from build123d import *

# Parameters (mm, degrees)
BOSS_EXTRUDE1_DEPTH = 6
SKETCH2_R           = 2.5
SKETCH2_R_2         = 12.5
SKETCH2_R_3         = 1.5
CUT_EXTRUDE1_DEPTH  = 96.876222287


with BuildPart() as part:
    # Sketch1 → Boss-Extrude1 (new body)
    with BuildSketch(Plane(origin=(0, 0, 0), x_dir=(1, 0, 0), z_dir=(0, 1, 0))):
        Polygon((0, 0), (-52.5, 0), (-52.5, 80), (52.5, 80), (52.5, 0), align=None)
    extrude(amount=BOSS_EXTRUDE1_DEPTH)

    # Sketch2 → Cut-Extrude1 (cut, through all)
    with BuildSketch(Plane(origin=(0, 6, 0), x_dir=(1, 0, 0), z_dir=(0, 1, 0))):
        with Locations(Location((-42.5, 70, 0), (0, 0, 270))):
            Circle(SKETCH2_R)
        with Locations(Location((42.5, 70, 0), (0, 0, 270))):
            Circle(SKETCH2_R)
        with Locations(Location((42.5, 10, 0), (0, 0, 270))):
            Circle(SKETCH2_R)
        with Locations(Location((0, 10, 0), (0, 0, 270))):
            Circle(SKETCH2_R)
        with Locations(Location((-42.5, 10, 0), (0, 0, 270))):
            Circle(SKETCH2_R)
        with Locations(Location((0, 41, 0), (0, 0, 270))):
            Circle(SKETCH2_R_2)
        with Locations(Location((-15.5, 56.5, 0), (0, 0, 270))):
            Circle(SKETCH2_R_3)
        with Locations(Location((15.5, 56.5, 0), (0, 0, 270))):
            Circle(SKETCH2_R_3)
        with Locations(Location((-15.5, 25.5, 0), (0, 0, 270))):
            Circle(SKETCH2_R_3)
        with Locations(Location((15.5, 25.5, 0), (0, 0, 270))):
            Circle(SKETCH2_R_3)
    extrude(amount=-CUT_EXTRUDE1_DEPTH, mode=Mode.SUBTRACT)


solid = part.part
Could you check a few things on this model? Use its own coordinates, in mm. Coordinates: 2 decimals unless noted, no trailing zeros. Write each loop counter-clockwise with the first axis right and the second up, starting at its lowest first coordinate (ties: lowest second). Pieces come first, ordered by that corner, then holes. Notation, with made-up numbers: (-3, 63.5) - (34, 63.5) arc R35 cw to (34, 95.5) - close; hole circle Ø1 at (62, 30.25). An arc over 180 degrees is marked (long way). Put each result on its own line as item: value. Start each with the question number.
Q1. Please list where these lines run through material, in increasing order: L1, parallel to X at y = 1.6, z = -56.5; L2, parallel to X at y = 4.5, z = -70.5; L3, parallel to X at y = 1.95, z = -45.
Q2. I want a section at B-B on x = 15.5. Write out the boundary of the cut face in (y, z), plus the area to 3 significant figures.
Q3. I want a section at C-C on y = 1.4. Count the separate pieces of the cut face and the enclosed holes in it, plus the area to 3 significant figures.
Q4. I want a section at D-D on z = -41. Write out the boundary of the cut face in (x, y), plus the area to 3 significant figures.
Q5. I'm going to push a flat-ended pin straight in: P1, Ø8, axis at x = 7, z = -38.5, coming from the +Y side. Where does the tip first touch, or does it pass through?
Q6. I want a section at A-A on z = -56.5. Write out the boundary of the cut face in (x, y).
Q7. Thinking about a two-plate mould opening in Z: for faces 1 (the flat face through (-1, 3, 0)), 2 (the flat face through (12, 6, -49)), 3 (the flat face through (-1, 3, -80)), 4 (the cylindrical face through (40.06, 3.04, -70.54)), which applies, pulls with the +Z half, pulls with the -Z half, needs draft (parallel to the pull), parting line crosses it, or undercut?
Checks:
1. L1: -52.5 to -17, -14 to 14, 17 to 52.5
1. L2: -52.5 to -44.95, -40.05 to 40.05, 44.95 to 52.5
1. L3: -52.5 to -11.84, 11.84 to 52.5
2. outline: (0, -80) - (6, -80) - (6, -58) - (0, -58) - close; (0, -55) - (6, -55) - (6, -27) - (0, -27) - close; (0, -24) - (6, -24) - (6, 0) - (0, 0) - close
2. area: 444 mm²
3. separate pieces: 1
3. enclosed holes: 10
3. area: 7,780 mm²
4. outline: (-52.5, 0) - (-12.5, 0) - (-12.5, 6) - (-52.5, 6) - close; (12.5, 0) - (52.5, 0) - (52.5, 6) - (12.5, 6) - close
4. area: 480 mm²
5. P1: through
6. outline: (-52.5, 0) - (-17, 0) - (-17, 6) - (-52.5, 6) - close; (-14, 0) - (14, 0) - (14, 6) - (-14, 6) - close; (17, 0) - (52.5, 0) - (52.5, 6) - (17, 6) - close
7. face 1: pulls with the +Z half
7. face 2: needs draft
7. face 3: pulls with the -Z half
7. face 4: undercut
